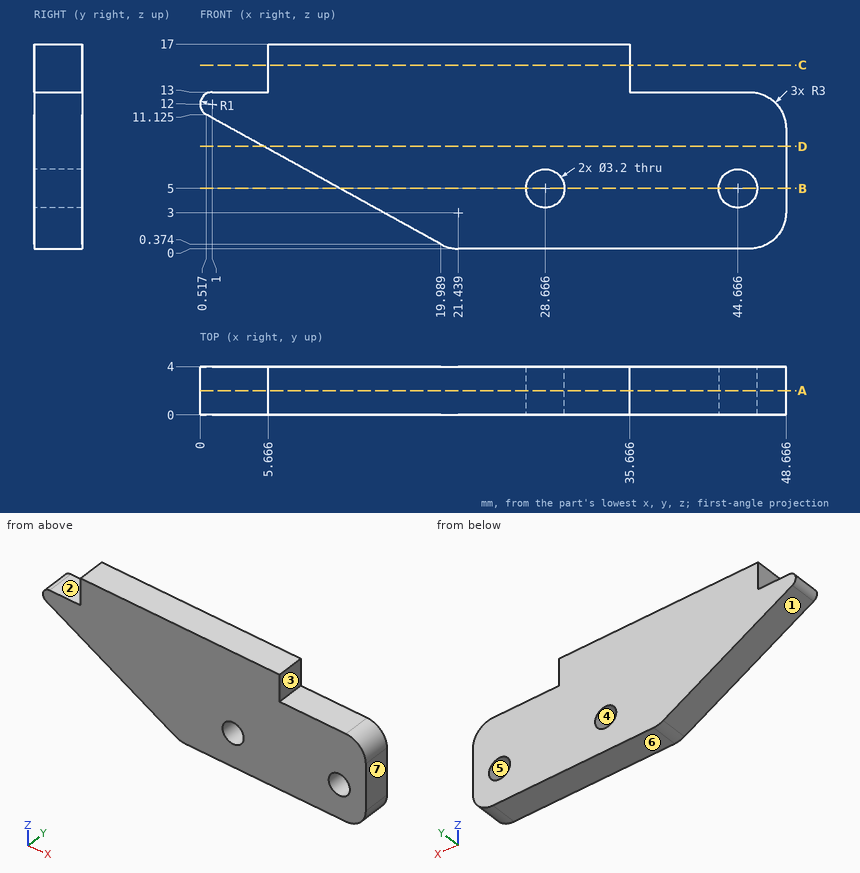
Study the drawing (mm; zero at the part's minimum x, y, z) and answer. A direction names the side the tool comes from. Give positions to 0.01 mm unless a question says otherwise; leave off trailing zeros. Loops run counter-clockwise (first coordinate to the right, second up) from the corner with the lowest first, then second, coordinate; pieces in that order, holes last. Notation, with made-up numbers: (44.25, -17.75) - (88.25, -17.75) arc R16 ccw to (88.25, 3.25) - close; hole circle Ø9 at (-36.5, -27.5). An arc over 180 degrees is marked (long way). Answer in a Markdown table with one row per item. Add a question column.
Q1. The part is cut by section D-D (z = 8.5). Determine the outline of the cut face in (x, y) (1 decimal).
Q2. The part is cut by section C-C (z = 15.25). Determine the outline of the cut face in (x, y) (1 decimal).
Q3. Consider line 1 along X through (y, z) = (1.7, 5) (1 decimal); line 2 along X through (y, z) = (3.1, 16) (1 decimal); line 3 along Z through (x, y) = (43.5, 1.05) (1 decimal). Determine where each line is inside the solid, lowest interval first.
Q4. Each of these flat-tipped pins is pushed along its axis until it touches: P1, Ø4, axis at x = 22.5, z = 5.5, coming from the -Y side; P2, Ø2, axis at x = 5, y = 1.5, coming from the -Z side; P3, Ø1, axis at x = 20, y = 3, coming from the -Z side; P4, Ø2, axis at y = 2, z = 16, coming from the -X side. Where does it stop, or does it pass through?
Q5. A tool of negligible diameter and unlimited length cuts with its end or side. For the marked faces 1, 2 and 3, from which of +Z, -Z, +X, -X, +Y, -Y can it reach the whole face along a straight path? Write none if from no direction.
Q6. Determine the mould class of the marked faces 4, 5, 6 and 7 for opening direction X: released by +X, released by -X, zero draft, split by the parting line, or undercut.
Q7. The part is cut by section B-B (z = 5). Determine the outline of the cut face in (x, y) (1 decimal).
Q8. The part is cut by section A-A (y = 2). Determine the outline of the cut face in (x, z) (1 decimal).
Solution:
| question | item | result |
|---|---|---|
| 1 | outline | (5.3, 0) - (48.7, 0) - (48.7, 4) - (5.3, 4) - close |
| 2 | outline | (5.7, 0) - (35.7, 0) - (35.7, 4) - (5.7, 4) - close |
| 3 | line 1 | x = 11.6 to 27.1, 30.3 to 43.1, 46.3 to 48.7 |
| 3 | line 2 | x = 5.7 to 35.7 |
| 3 | line 3 | z = 0 to 3.9, 6.1 to 13 |
| 4 | P1 | stops at y = 0 |
| 4 | P2 | stops at z = 8.1 |
| 4 | P3 | stops at z = 0.15 |
| 4 | P4 | stops at x = 5.67 |
| 5 | face 1 | -Z, -X, +Y, -Y |
| 5 | face 2 | +Z, -X, +Y, -Y |
| 5 | face 3 | +Z, +X, +Y, -Y |
| 6 | face 4 | undercut |
| 6 | face 5 | undercut |
| 6 | face 6 | zero draft |
| 6 | face 7 | released by +X |
| 7 | outline | (11.6, 0) - (27.1, 0) - (27.1, 4) - (11.6, 4) - close; (30.3, 0) - (43.1, 0) - (43.1, 4) - (30.3, 4) - close; (46.3, 0) - (48.7, 0) - (48.7, 4) - (46.3, 4) - close |
| 8 | outline | (0.5, 11.1) - (20, 0.4) arc R3 ccw to (21.4, 0) - (45.7, 0) arc R3 ccw to (48.7, 3) - (48.7, 10) arc R3 ccw to (45.7, 13) - (35.7, 13) - (35.7, 17) - (5.7, 17) - (5.7, 13) - (1, 13) arc R1 ccw to start; hole circle Ø3.2 at (28.7, 5); hole circle Ø3.2 at (44.7, 5) |
